from build123d import *

# Parameters (mm, degrees)
F0_W            = 50.8
F0_H            = 50.8
F0_R            = 25.4
F1_DEPTH        = 25.4
F2_R            = 12.7
F4_D            = 10.16
F4_COPIES_COUNT = 6
F5_DEPTH        = 25.401
F5_TAPER        = 10


# Not quite as in the source:
# - a pattern or mirror of a feature is missing from the dataset's text; its kind, count and spacing are read off the source's solid


with BuildPart() as f1:
    # F0 (on Top) → F1 (new body)
    with BuildSketch(Plane.XY):
        with Locations((88.9, 0)):
            Rectangle(F0_W, F0_H)
        Polygon((63.5, 25.4), (63.5, 76.2), (-63.5, 76.2), (-63.5, -76.2), (63.5, -76.2), (63.5, -25.4), align=None)
        Circle(F0_R, mode=Mode.SUBTRACT)
    extrude(amount=F1_DEPTH)

    # F2
    f2_edges = [f1.edges().sort_by_distance(p)[0] for p in [
        (63.5, -25.4, 12.7),
        (63.5, 25.4, 12.7),
        (114.3, -25.4, 12.7),
        (114.3, 25.4, 12.7),
    ]]
    fillet(f2_edges, radius=F2_R)

    # F4 (through all)
    with Locations(Plane.XY.offset(25.4)):
        with Locations((0, -50.8)):
            f4 = Hole(F4_D / 2)

    # F4_copies: F4 ×6 about axis
    f4_copies_axis = Axis((0, 0, 0), (0, 0, 1))
    for i in range(1, F4_COPIES_COUNT):
        add(f4.rotate(f4_copies_axis, i * 360 / F4_COPIES_COUNT), mode=Mode.SUBTRACT)

    # F3 (on face) → F5 (cut, through all)
    with BuildSketch(Plane.XY.offset(25.4)):
        with BuildLine():
            ThreePointArc((107.9500002354, 12.7), (106.090128227, 17.190128227), (101.6, 19.0500002354))
            Line((101.6, 19.0500002354), (76.2000002354, 19.0500002354))
            ThreePointArc((76.2000002354, 19.0500002354), (71.7098721749, 17.190128296), (69.8500002354, 12.7000002354))
            Line((69.8500002354, 12.7000002354), (69.8500002354, -12.7000002354))
            ThreePointArc((69.8500002354, -12.7000002354), (71.7098721749, -17.190128296), (76.2000002354, -19.0500002354))
            Line((76.2000002354, -19.0500002354), (101.6, -19.0500002354))
            ThreePointArc((101.6, -19.0500002354), (106.090128227, -17.190128227), (107.9500002354, -12.7))
            Line((107.9500002354, -12.7), (107.9500002354, 12.7))
        make_face()
    extrude(amount=-F5_DEPTH, taper=F5_TAPER, mode=Mode.SUBTRACT)

    # F6: F1 across face


with BuildPart() as f1_1:
    add(f1.part)
    add(f1.part.mirror(Plane(origin=(-63.5, 0, 12.7), x_dir=(0, -1, 0), z_dir=(-1, 0, 0))))


solid = f1_1.part
Read the model definition and answer for the solid it produces. Units are mm, in the model's axes. A direction names the side the tool comes from. Give positions to 0.01 mm unless a question says otherwise; leave off trailing zeros. Write each loop counter-clockwise with the first axis right and the second up, starting at its lowest first coordinate (ties: lowest second). Pieces come first, ordered by that corner, then holes. Notation, with made-up numbers: (81.5, 44) - (85.5, 44) arc R23 cw to (85.5, 71) - close; hole circle Ø11 at (34.25, -18.5). An arc over 180 degrees is marked (long way). Use CSV: the item, a comma, the result in double quotes. Start each with the question number.
(1) For faces 4 (the flat face through (-190.5, 57, 13)), 5 (the flat face through (-61, 1, 0)), 6 (the flat face through (63.5, -57, 13)), 7 (the conical face through (73.35, 15.62, 12.52)), determine the directions among +Z, -Z, +X, -X, +Y, -Y from which every point of the face is accessible in a straight line to the end or side of a thin tool.
(2) Find section B-B (x = -146). Give the vertices of the cut face in (y, z), plus the area to 3 significant figures.
(3) Find section A-A (y = 50.8). Give the vertices of the cut face in (x, z), plus the area to 3 significant figures.
(4) Given P1, Ø6, axis at y = 16, z = 3.5, coming from the -X side; P2, Ø6, axis at y = -39.5, z = 20.5, coming from the +X side; P3, Ø12.5, axis at x = -212.5, z = 12, coming from the +Y side; P4, Ø6, axis at x = 0, y = 50.8, coming from the +Z side, each flat-ended and moving along its own axis, determine where each tip first touches the part or whether it passes through.
(5) Consider line 1 along Y through (x, z) = (0, 19.75); line 2 along Y through (x, z) = (-82.5, 23); line 3 along X through (y, z) = (9.5, 23.5). Determine where each line is inside the solid, lowest interval first.
(6) Find section C-C (y = 0). Count the separate pieces of the cut face and the enclosed holes in it, plus the area to 3 significant figures.
(7) Determine the mould class of faces 1 (the cylindrical face through (67.32, 29.02, 12.88)), 2 (the flat face through (89, -25.4, 13)), 3 (the conical face through (73.28, -15.55, 12.52)) for opening direction X: +X half, -X half, draft (parallel to the pull), parting line (faces both ways), or undercut.
Findings below:
1,face 4,"+Z, -Z, -X, +Y"
1,face 5,"-Z, +X, -X, +Y, -Y"
1,face 6,"+Z, -Z, +X, -Y"
1,face 7,"+Z"
2,outline,"(-76.2, 0) - (-16.86, 0) - (-16.86, 25.4) - (-76.2, 25.4) - close; (16.86, 0) - (76.2, 0) - (76.2, 25.4) - (16.86, 25.4) - close"
2,area,"3,010 mm2"
3,outline,"(-190.5, 0) - (-132.08, 0) - (-132.08, 25.4) - (-190.5, 25.4) - close; (-121.92, 0) - (-5.08, 0) - (-5.08, 25.4) - (-121.92, 25.4) - close; (5.08, 0) - (63.5, 0) - (63.5, 25.4) - (5.08, 25.4) - close"
3,area,"5,940 mm2"
4,P1,"x = -241.3"
4,P2,"x = 63.6"
4,P3,"y = 25.4"
4,P4,"through"
5,line 1,"-76.2 to -55.88, -45.72 to -25.4, 25.4 to 45.72, 55.88 to 76.2"
5,line 2,"-76.2 to -30.45, -20.35 to 20.35, 30.45 to 76.2"
5,line 3,"-241.3 to -234.61, -197.19 to -150.56, -103.44 to -23.56, 23.56 to 70.19, 107.61 to 114.3"
6,separate pieces,"5"
6,enclosed holes,"0"
6,area,"4,740 mm2"
7,face 1,"+X half"
7,face 2,"draft"
7,face 3,"undercut"
